Build history of the part. All positions in model axes, mm. Coordinates: 2 decimals unless noted, no trailing zeros. Order: outer loops, then holes, each group sorted by start corner. A loop starts at its lowest first (then second) coordinate and runs counter-clockwise, first axis right, second up. Notation, with made-up numbers: M 56.25,79 L 74.25,79 A29 cw 74.25,101 Z; hole C -4.5,-25 d1. An arc over 180 degrees is marked long. Write item = value, one per line. Start each with the question number.
Q1. Band-saw the part on B-B on y = 299.8. Write the cut outline in (x, z), plus the area to 3 significant figures.
Q2. Band-saw the part on A-A on z = 1. Write the cut outline in (x, y), plus the area to 3 significant figures.
Q3. Band-saw the part on C-C on x = 4. Write the cut outline in (y, z).
Q4. Pin check, flat tips, straight feed: P1, Ø2, axis at x = -162, z = 1, coming from the +Y side; P2, Ø1, axis at y = 284.5, z = 2, coming from the +X side; P3, Ø2.5, axis at x = 4, y = 299.8, coming from the +Z side. Stop position of each tip, or through.
Q5. Band-saw the part on D-D on y = 250. Write the cut outline in (x, z).
Q6. Drill centre lines: probe 1 along Y at (x, z) = (4, 1.9); probe 2 along X at (y, z) = (299.8, 3.15); probe 3 along X at (y, z) = (145.5, 3). Where is each one in solid material? Low to high.
```python
from build123d import *

# Parameters (mm, degrees)
BOSS_EXTRUDE1_DEPTH = 4.6
SKETCH2_R           = 2.25
CUT_EXTRUDE1_DEPTH  = 362.31293858


with BuildPart() as part:
    # Sketch1 → Boss-Extrude1 (new body)
    with BuildSketch(Plane.XY):
        with BuildLine():
            Line((6.553588095, 296.721171027), (-3.221693894, 288.613528827))
            Line((-3.221693894, 288.613528827), (-1.721460888, 286.804716805))
            Line((-1.721460888, 286.804716805), (-187.42097357, 132.785097993))
            Line((-187.42097357, 132.785097993), (-195.528615771, 142.560379981))
            Line((-195.528615771, 142.560379981), (-9.829103088, 296.579998794))
            Line((-9.829103088, 296.579998794), (-8.328870083, 294.771186772))
            Line((-8.328870083, 294.771186772), (1.446411905, 302.878828973))
            ThreePointArc((1.446411905, 302.878828973), (7.078828973, 302.353588095), (6.553588095, 296.721171027))
        make_face()
    extrude(amount=BOSS_EXTRUDE1_DEPTH)

    # Sketch2 → Cut-Extrude1 (cut, through all)
    with BuildSketch(Plane.XY.offset(4.6)):
        with Locations((4, 299.8)):
            Circle(SKETCH2_R)
    extrude(amount=-CUT_EXTRUDE1_DEPTH, mode=Mode.SUBTRACT)


solid = part.part
```
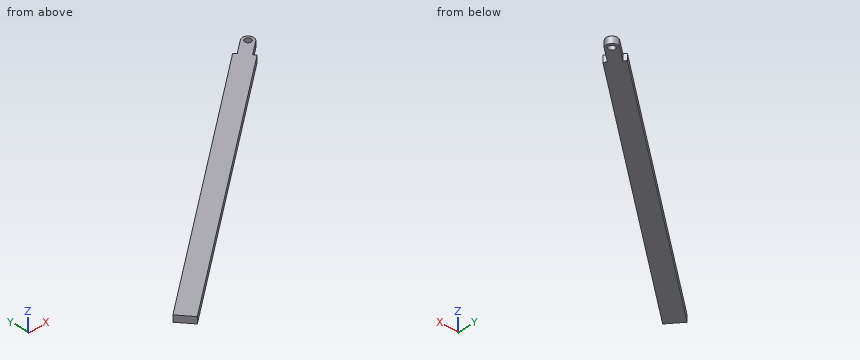
Recorded:
q1.outline = M -2.27,0 L 1.75,0 L 1.75,4.6 L -2.27,4.6 Z; M 6.25,0 L 8,0 L 8,4.6 L 6.25,4.6 Z
q1.area = 26.5 mm2
q2.outline = M -195.53,142.56 L -187.42,132.79 L -1.72,286.8 L -3.22,288.61 L 6.55,296.72 A4 ccw 1.45,302.88 L -8.33,294.77 L -9.83,296.58 Z; hole C 4,299.8 d4.5
q2.area = 3,170 mm2
q3.outline = M 294.6,0 L 297.55,0 L 297.55,4.6 L 294.6,4.6 Z; M 302.05,0 L 303.8,0 L 303.8,4.6 L 302.05,4.6 Z
q4.P1 = 171.2
q4.P2 = -3.9
q4.P3 = through
q5.outline = M -65.99,0 L -46.1,0 L -46.1,4.6 L -65.99,4.6 Z
q6.probe_1 = 294.6 to 297.55, 302.05 to 303.8
q6.probe_2 = -2.27 to 1.75, 6.25 to 8
q6.probe_3 = -191.98 to -172.09
